Part model, mm, in its own coordinate system. Coordinates: 2 decimals unless noted, no trailing zeros. Loops run counter-clockwise (first coordinate to the right, second up) from the corner with the lowest first, then second, coordinate; pieces in that order, holes last.
Autodesk Inventor part; units mm, degrees
ref_plane "YZ Plane" through (0, 0, 0) normal (1, 0, 0) x (0, 1, 0)
ref_plane "XZ Plane" through (0, 0, 0) normal (0, 1, 0) x (-1, 0, 0)
ref_plane "XY Plane" through (0, 0, 0) normal (0, 0, 1) x (1, 0, 0)
sketch "Sketch1" plane through (0, 0, 0) normal (0, 1, 0) x (-1, 0, 0)
  line L0 (-3.5, -2.0207) -> (-3.5, 2.0207)
  line L1 (-3.5, 2.0207) -> (0, 4.0415)
  line L2 (0, 4.0415) -> (3.5, 2.0207)
  line L3 (3.5, 2.0207) -> (3.5, -2.0207)
  line L4 (3.5, -2.0207) -> (0, -4.0415)
  line L5 (0, -4.0415) -> (-3.5, -2.0207)
  point P0 (0, 0)
  point P1 (0, 0)
  dimension "d0" = 7
extrude "Extrusion1" add sketch "Sketch1" against normal blind 16
chamfer "Chamfer1" distance 0.1 angle 45 12 edges at (-1.75, -16, 3.0311) (1.75, -16, 3.0311) (3.5, -16, 0) (1.75, -16, -3.0311) (-1.75, -16, -3.0311) (-3.5, -16, 0) (1.75, 0, 3.0311) (-1.75, 0, 3.0311) (-3.5, 0, 0) (-1.75, 0, -3.0311) (1.75, 0, -3.0311) (3.5, 0, 0)
sketch "Sketch2" plane through (0, -16, 0) normal (0, -1, 0) x (1, 0, 0)
  circle A0 centre (0, 0) radius 2
  dimension "d6" = 4
extrude "Extrusion2" cut sketch "Sketch2" against normal through all
chamfer "Chamfer2" distance 0.2 angle 45 2 edges at (-2, -16, 0) (-2, 0, 0)
thread "Thread1"
properties part number "09-0003" material "Aluminum 6061"
Q1. Saw through at B-B (y = -7.5). List the corners of the cut face in (x, z), plus the area to 3 significant figures.
Q2. Drop flat-ended pins along their axis: P1, Ø3, axis at x = -2, y = -14, coming from the +Z side; P2, Ø3, axis at x = 2, y = -5.5, coming from the -Z side. Give the stop position or say it passes through.
Q3. Saw through at A-A (z = 0). List the corners of the cut face in (x, y).
Q4. Saw through at D-D (x = 2.75). List the corners of the cut face in (y, z), plus the area to 3 significant figures.
Q5. Saw through at C-C (z = -3.5). List the corners of the cut face in (x, y), plus the area to 3 significant figures.
Q6. Mould opens along Z. For faces 1 (the flat face through (1.8, -7.9, 3)), 2 (the cylindrical face through (0, -8, -2)), 3 (the flat face through (-1.8, -7.9, -3)), 4 (the flat face through (3.5, -8, 0)) say: released by +Z, released by -Z, zero draft, split by the parting line, or undercut.
Q7. Probe line 1 (Z direction, x = 0.5, y = -4.5); line 2 (Z direction, x = 0.75, y = -2.5); line 3 (X direction, y = -15.5, z = -1). List the from-to ranges inside material, lowest first.
Checked values:
1. outline: (-3.5, -2.02) - (0, -4.04) - (3.5, -2.02) - (3.5, 2.02) - (0, 4.04) - (-3.5, 2.02) - close; hole circle Ø4 at (0, 0)
1. area: 29.9 mm2
2. P1: stops at z = 3.75
2. P2: stops at z = -3.75
3. outline: (-3.5, -15.9) - (-3.4, -16) - (-2.2, -16) - (-2, -15.8) - (-2, -0.2) - (-2.2, 0) - (-3.4, 0) - (-3.5, -0.1) - close; (2, -15.8) - (2.2, -16) - (3.4, -16) - (3.5, -15.9) - (3.5, -0.1) - (3.4, 0) - (2.2, 0) - (2, -0.2) - close
4. outline: (-16, -2.34) - (-15.9, -2.45) - (-0.1, -2.45) - (0, -2.34) - (0, 2.34) - (-0.1, 2.45) - (-15.9, 2.45) - (-16, 2.34) - close
4. area: 78.5 mm2
5. outline: (-0.94, -15.9) - (-0.74, -16) - (0.74, -16) - (0.94, -15.9) - (0.94, -0.1) - (0.74, 0) - (-0.74, 0) - (-0.94, -0.1) - close
5. area: 30.0 mm2
6. face 1: released by +Z
6. face 2: undercut
6. face 3: released by -Z
6. face 4: zero draft
7. line 1: z = -3.75 to -1.94, 1.94 to 3.75
7. line 2: z = -3.61 to -1.85, 1.85 to 3.61
7. line 3: x = -3.5 to -1.73, 1.73 to 3.5
